Geometry: final body of the model. Coordinates: model frame, mm. A direction names the side the tool comes from. Give positions to 0.01 mm unless a question says otherwise; leave off trailing zeros. Loops run counter-clockwise (first coordinate to the right, second up) from the corner with the lowest first, then second, coordinate; pieces in that order, holes last.
from build123d import *

# Parameters (mm, degrees)
ESBO_O1_W                = 126.9
ESBO_O1_H                = 38.1
RESSALTO_EXTRUS_O2_DEPTH = 3.9
ESBO_O3_W                = 6.5
ESBO_O3_H                = 38.1
RESSALTO_EXTRUS_O3_DEPTH = 53.1
ESBO_O4_W                = 25.3
ESBO_O4_H                = 25.3
ESBO_O4_R                = 3.2
CORTE_EXTRUS_O1_DEPTH    = 4
CORTE_EXTRUS_O2_DEPTH    = 50
CORTE_EXTRUS_O3_DEPTH    = 5.65
ESBO_O9_R                = 2.5
CORTE_EXTRUS_O4_DEPTH    = 10


with BuildPart() as part:
    # Esboço1 → Ressalto-extrusão2 (new body)
    with BuildSketch(Plane.XY):
        with Locations((-63.45, 19.05)):
            Rectangle(ESBO_O1_W, ESBO_O1_H)
    extrude(amount=RESSALTO_EXTRUS_O2_DEPTH)

    # Esboço3 → Ressalto-extrusão3 (add)
    with BuildSketch(Plane.XY.offset(3.9)):
        with Locations((-123.65, 19.05)):
            Rectangle(ESBO_O3_W, ESBO_O3_H)
        with Locations((-3.25, 19.05)):
            Rectangle(ESBO_O3_W, ESBO_O3_H)
    extrude(amount=RESSALTO_EXTRUS_O3_DEPTH)

    # Esboço4 → Corte-extrusão1 (cut)
    with BuildSketch(Plane.ZY.offset(126.9)):
        with Locations((38.65, 19.05)):
            Rectangle(ESBO_O4_W, ESBO_O4_H)
        with Locations((38.65, 19.05)):
            Circle(ESBO_O4_R, mode=Mode.SUBTRACT)
    extrude(amount=-CORTE_EXTRUS_O1_DEPTH, mode=Mode.SUBTRACT)

    # Esboço6 → Corte-extrusão2 (cut)
    with BuildSketch(Plane.ZY.offset(126.9)):
        with BuildLine():
            Line((38.65, 22.25), (57, 22.25))
            Line((57, 22.25), (57, 15.85))
            Line((57, 15.85), (38.65, 15.85))
            ThreePointArc((38.65, 15.85), (35.45, 19.05), (38.65, 22.25))
        make_face()
    extrude(amount=-CORTE_EXTRUS_O2_DEPTH, mode=Mode.SUBTRACT)

    # Esboço7 → Corte-extrusão3 (cut)
    with BuildSketch(Plane(origin=(0, 0, 0), x_dir=(0, 0, -1), z_dir=(1, 0, 0))):
        with BuildLine():
            Line((-3.5, 14.7), (0, 14.7))
            Line((0, 14.7), (0, 23.4))
            Line((0, 23.4), (-3.5, 23.4))
            ThreePointArc((-3.5, 23.4), (-7.85, 19.05), (-3.5, 14.7))
        make_face()
    extrude(amount=-CORTE_EXTRUS_O3_DEPTH, mode=Mode.SUBTRACT)

    # Esboço9 → Corte-extrusão4 (cut)
    with BuildSketch(Plane(origin=(0, 0, 0), x_dir=(0, 0, -1), z_dir=(1, 0, 0))):
        with Locations((-53.5, 19.05)):
            Circle(ESBO_O9_R)
    extrude(amount=-CORTE_EXTRUS_O4_DEPTH, mode=Mode.SUBTRACT)


solid = part.part
Item 1: Section query D-D on y = 10. Return loops of the section in (x, z).
Values follow:
outline: (-126.9, 0) - (0, 0) - (0, 57) - (-6.5, 57) - (-6.5, 3.9) - (-120.4, 3.9) - (-120.4, 57) - (-126.9, 57) - (-126.9, 51.3) - (-122.9, 51.3) - (-122.9, 26) - (-126.9, 26) - close
Item 2: Section query A-A on z = 14. Return loops of the section in (x, y).
Values follow:
outline: (-126.9, 0) - (-120.4, 0) - (-120.4, 38.1) - (-126.9, 38.1) - close; (-6.5, 0) - (0, 0) - (0, 38.1) - (-6.5, 38.1) - close
Item 3: Ray query, probe 1 along Z at (x, y) = (-2, 19); probe 2 along Y at (x, z) = (-2, 53.5); probe 3 along X at (y, z) = (32, 9.5). Return the intervals inside material, ascending.
Values follow:
probe 1: z = 7.85 to 51, 56 to 57
probe 2: y = 0 to 16.55, 21.55 to 38.1
probe 3: x = -126.9 to -120.4, -6.5 to 0
Item 4: Pin query (flat end, axial travel): pin 1 (11.5 mm diameter, centred on x = -85, y = 18.5, fed in from +Z). Return the tip coordinate at first contact, or that it passes through.
Values follow:
pin 1: stops at z = 3.9
Item 5: Section query C-C on z = 53.5. Return loops of the section in (x, y).
Values follow:
outline: (-126.9, 0) - (-120.4, 0) - (-120.4, 15.85) - (-126.9, 15.85) - close; (-126.9, 22.25) - (-120.4, 22.25) - (-120.4, 38.1) - (-126.9, 38.1) - close; (-6.5, 0) - (0, 0) - (0, 16.55) - (-6.5, 16.55) - close; (-6.5, 21.55) - (0, 21.55) - (0, 38.1) - (-6.5, 38.1) - close
Item 6: Set-up query: faces 1 (the face through (-122, 22.25, 50)), 2 (the face through (-6.5, 19, 30)), 3 (the face through (-125, 6.4, 38)), 4 (the face through (-3.2, 18.09, 51.19)). Return all of +Z, -Z, +X, -X, +Y, -Y with unobstructed straight access to the full face (end or side cutting, diameter ignored); none if empty.
Values follow:
face 1: +Z, -X
face 2: +Z, +Y, -Y
face 3: -X
face 4: +X, -X
Item 7: Section query B-B on y = 19.05. Return loops of the section in (x, z).
Values follow:
outline: (-126.9, 0) - (-5.65, 0) - (-5.65, 7.85) - (0, 7.85) - (0, 51) - (-6.5, 51) - (-6.5, 3.9) - (-120.4, 3.9) - (-120.4, 35.45) - (-122.9, 35.45) - (-122.9, 26) - (-126.9, 26) - close; (-6.5, 56) - (0, 56) - (0, 57) - (-6.5, 57) - close
Item 8: Draft query along X for faces 5 (the face through (-120.4, 19, 30)), 6 (the face through (-122, 15.85, 50)), 7 (the face through (-122.9, 16, 36)), 8 (the face through (-5.65, 19, 4)). Return one class per face: +X half, -X half, draft (parallel to the pull), parting line (faces both ways), or undercut.
Values follow:
face 5: undercut
face 6: draft
face 7: -X half
face 8: +X half
